Input: dimensioned drawing with shaded views. Units: mm. Origin: part minimum x, y, z. Round coordinates to 2 decimals unless told otherwise and drop trailing zeros. Loops run counter-clockwise (first coordinate to the right, second up) from the corner with the lowest first, then second, coordinate; pieces in that order, holes last. Notation, with made-up numbers: (69, -9.5) - (84, -9.5) arc R31 ccw to (84, 25.5) - close; hole circle Ø7 at (14, -21.75). An arc over 180 degrees is marked (long way). One line per question, with ' | ' between items. Start each with the question number.
1. Pin query (flat end, axial travel): pin 1 (5 mm diameter, centred on y = 4, z = 16, fed in from +X); pin 2 (0.6 mm diameter, centred on x = 7, y = 15, fed in from -Z); pin 3 (4.5 mm diameter, centred on x = 7, z = 9.5, fed in from +Y); pin 4 (1.5 mm diameter, centred on x = 9.5, y = 2.5, fed in from -Z). Return the tip coordinate at first contact, or that it passes through.
2. Cut plane B-B (z = 36.5). Return loops of the section in (x, y).
3. Ray query, line 1 (X direction, y = 11.25, z = 32.5); line 2 (X direction, y = 13.75, z = 20.5); line 3 (X direction, y = 14.25, z = 2). Return the intervals inside material, ascending.
4. Cut plane C-C (z = 19.5). Return loops of the section in (x, y), then the cut area to 3 significant figures.
5. Cut plane A-A (x = 7.5). Return loops of the section in (y, z).
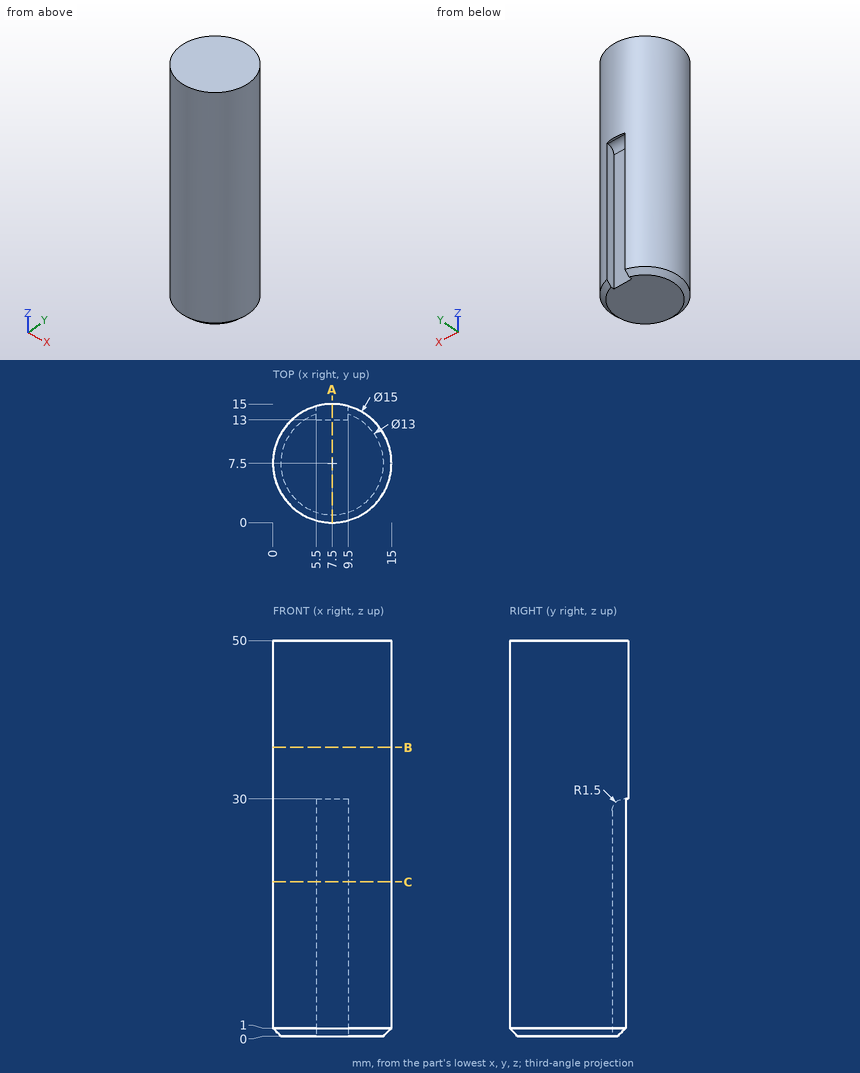
Answers follow:
1) pin 1: stops at x = 14.93 | pin 2: stops at z = 30 | pin 3: stops at y = 14.73 | pin 4: stops at z = 0
2) outline: circle Ø15 at (7.5, 7.5)
3) line 1: x = 1 to 14 | line 2: x = 3.35 to 5.5, 9.5 to 11.65 | line 3: x = 4.23 to 5.5, 9.5 to 10.77
4) outline: (5.5, 13) - (5.5, 14.73) arc R7.5 ccw (long way) to (9.5, 14.73) - (9.5, 13) - close | area: 169 mm2
5) outline: (0, 1) - (1, 0) - (13, 0) - (13, 28.5) arc R1.5 cw to (14.5, 30) - (15, 30) - (15, 50) - (0, 50) - close
